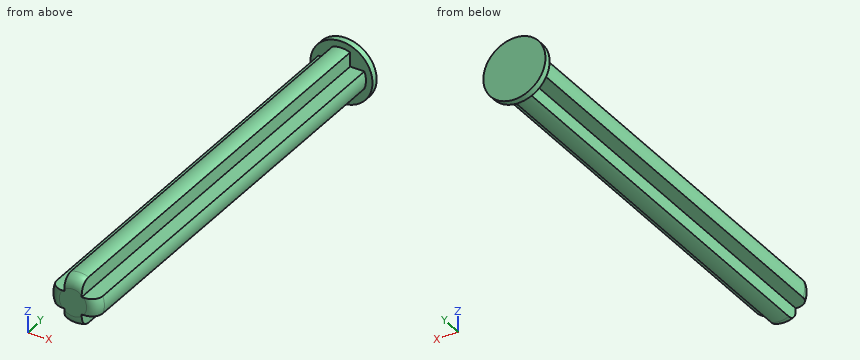
from build123d import *

# Parameters (mm, degrees)
BOSS_EXTRUDE1_DEPTH = 39.4
FILLET1_R           = 1
FILLET2_R           = 1
FILLET3_R           = 1
FILLET4_R           = 1
SKETCH3_R           = 2.85
BOSS_EXTRUDE2_DEPTH = 0.6


with BuildPart() as part:
    # Sketch1 → Boss-Extrude1 (new body)
    with BuildSketch(Plane(origin=(0, 0, 0), x_dir=(1, 0, 0), z_dir=(0, 1, 0))):
        with BuildLine():
            Line((-0.8, -0.8), (-0.8, -2.102974084))
            ThreePointArc((-0.8, -2.102974084), (0, -2.25), (0.8, -2.102974084))
            Line((0.8, -2.102974084), (0.8, -0.8))
            Line((0.8, -0.8), (2.102974084, -0.8))
            ThreePointArc((2.102974084, -0.8), (2.25, 0), (2.102974084, 0.8))
            Line((2.102974084, 0.8), (0.8, 0.8))
            Line((0.8, 0.8), (0.8, 2.102974084))
            ThreePointArc((0.8, 2.102974084), (0, 2.25), (-0.8, 2.102974084))
            Line((-0.8, 2.102974084), (-0.8, 0.8))
            Line((-0.8, 0.8), (-2.102974084, 0.8))
            ThreePointArc((-2.102974084, 0.8), (-2.25, 0), (-2.102974084, -0.8))
            Line((-2.102974084, -0.8), (-0.8, -0.8))
        make_face()
    extrude(amount=BOSS_EXTRUDE1_DEPTH)

    # Fillet1
    fillet1_edges = [part.edges().sort_by_distance(p)[0] for p in [
        (-2.25, 0, 0),
    ]]
    fillet(fillet1_edges, radius=FILLET1_R)

    # Fillet2
    fillet2_edges = [part.edges().sort_by_distance(p)[0] for p in [
        (0, 0, 2.25),
    ]]
    fillet(fillet2_edges, radius=FILLET2_R)

    # Fillet3
    fillet3_edges = [part.edges().sort_by_distance(p)[0] for p in [
        (2.25, 0, 0),
    ]]
    fillet(fillet3_edges, radius=FILLET3_R)

    # Fillet4
    fillet4_edges = [part.edges().sort_by_distance(p)[0] for p in [
        (0, 0, -2.25),
    ]]
    fillet(fillet4_edges, radius=FILLET4_R)

    # Sketch3 → Boss-Extrude2 (add)
    with BuildSketch(Plane(origin=(0, 39.4, 0), x_dir=(1, 0, 0), z_dir=(0, 1, 0))):
        with Locations(Location((0, 0, 0), (0, 0, 270))):
            Circle(SKETCH3_R)
    extrude(amount=-BOSS_EXTRUDE2_DEPTH)


solid = part.part
The listing builds one solid part. Answer for the finished solid, in the listing's coordinates (mm). Coordinates: 2 decimals unless noted, no trailing zeros. Write each loop counter-clockwise with the first axis right and the second up, starting at its lowest first coordinate (ties: lowest second). Pieces come first, ordered by that corner, then holes. Notation, with made-up numbers: M 25,-13.5 L 39,-13.5 A38 ccw 39,24.5 Z; hole C 2,18.25 d6. An arc over 180 degrees is marked long. Put each result on its own line as item: value. Start each with the question number.
1. A cutting plane is placed at C-C on z = 0. Write down the section's boundary in (x, y).
2. A cutting plane is placed at B-B on y = 34.5. Write down the section's boundary in (x, z), then the cut area to 3 significant figures.
3. Flat-ended cylindrical pins translate along their axes: P1, Ø2, axis at x = -0.5, y = 8.5, coming from the -Z side; P2, Ø0.7, axis at y = 10.5, z = 1.5, coming from the +X side; P3, Ø1, axis at x = -1.5, y = 18.5, coming from the -Z side. Find the tip coordinate at first contact, or state that the pin passes through.
4. Consider line 1 (Z direction, x = -1.4, y = 18.5); line 2 (Y direction, x = -1.5, z = 2.2). Determine where each line is inside the solid, lowest interval first. Write a range as from..to.
5. A cutting plane is placed at A-A on x = 0. Write down the section's boundary in (y, z), then the cut area to 3 significant figures.
Resolved:
1. outline: M -2.85,38.8 L -2.25,38.8 L -2.25,1 A1 ccw -1.25,0 L 1.25,0 A1 ccw 2.25,1 L 2.25,38.8 L 2.85,38.8 L 2.85,39.4 L -2.85,39.4 Z
2. outline: M -2.1,-0.8 L -0.8,-0.8 L -0.8,-2.1 A2.25 ccw 0.8,-2.1 L 0.8,-0.8 L 2.1,-0.8 A2.25 ccw 2.1,0.8 L 0.8,0.8 L 0.8,2.1 A2.25 ccw -0.8,2.1 L -0.8,0.8 L -2.1,0.8 A2.25 ccw Z
2. area: 11.5 mm2
3. P1: stops at z = -2.25
3. P2: stops at x = 0.8
3. P3: stops at z = -0.8
4. line 1: z = -0.8..0.8
4. line 2: y = 38.8..39.4
5. outline: M 0,-1.25 A1 ccw 1,-2.25 L 38.8,-2.25 L 38.8,-2.85 L 39.4,-2.85 L 39.4,2.85 L 38.8,2.85 L 38.8,2.25 L 1,2.25 A1 ccw 0,1.25 Z
5. area: 178 mm2
